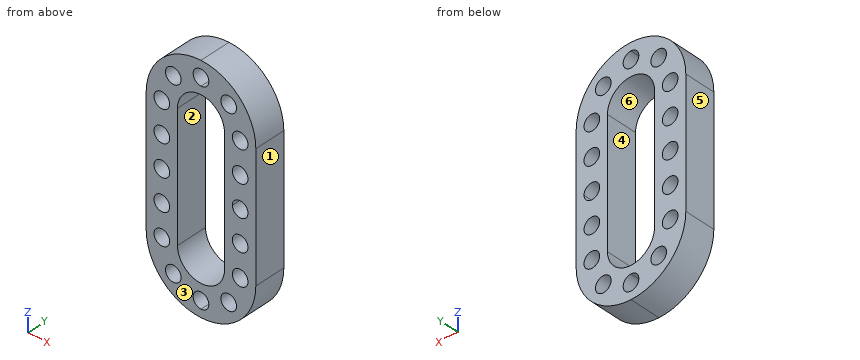
```python
from build123d import *
from build123d import SkipClean  # not in build123d's __all__

# Parameters (mm, degrees)
F0_R     = 5
F1_DEPTH = 20


with BuildPart() as f1:
    # F0 (on Front) → F1 (new body)
    with BuildSketch(Plane.XZ):
        with BuildLine():
            ThreePointArc((-15, 40), (-10.6066017178, 50.6066017178), (0, 55))
            Line((0, 55), (0.0401919294, 60.0001615417))
            ThreePointArc((0.0401919294, 60.0001615417), (-4.9999596144, 64.979903873), (0, 70))
            Line((0, 70), (0, 75))
            ThreePointArc((0, 75), (-24.7487373415, 64.7487373415), (-35, 40))
            Line((-35, 40), (-35, 0))
            Line((-35, 0), (-30, 0))
            ThreePointArc((-30, 0), (-25, 5), (-20, 0))
            Line((-20, 0), (-15, 0))
            Line((-15, 0), (-15, 40))
        make_face()
        with Locations((-25, 20)):
            Circle(F0_R, mode=Mode.SUBTRACT)
        with Locations((-25, 40)):
            Circle(F0_R, mode=Mode.SUBTRACT)
        with Locations((-17.6776695297, 57.6776695297)):
            Circle(F0_R, mode=Mode.SUBTRACT)
    extrude(amount=F1_DEPTH)

    # F2: F1 across plane


with BuildPart() as f1_1:
    add(f1.part, clean=False)
    add(f1.part.mirror(Plane.YZ), clean=False)

    # F3: F1 across plane


with BuildPart() as f1_2:
    add(f1_1.part, clean=False)
    with SkipClean():  # cleaning this boolean's faces spoils the solid; the shape is the same uncleaned
        add(f1_1.part.mirror(Plane.XY), clean=False)


solid = f1_2.part
```
For this review, take the finished solid that the model builds, in its own axes (mm). Face numbers are marked on the shaded views. A direction names the side the tool comes from. Round coordinates to 2 decimals unless told otherwise and drop trailing zeros. Order: outer loops, then holes, each group sorted by start corner. A loop starts at its lowest first (then second) coordinate and runs counter-clockwise, first axis right, second up. Notation, with made-up numbers: (18, 48.5) -> (73, 48.5) arc R9 ccw to (73, 62.5) -> close; hole circle Ø4 at (-12.75, -28). An arc over 180 degrees is marked (long way). Use a Markdown table: item, result.
Item 1: Draft analysis for pull direction X (two halves, no side actions). For the marked faces 1, 2, 3 and 4, state which applies: +X half, -X half, draft (parallel to the pull), parting line (faces both ways), or undercut.
Resolved:
| item | result |
|---|---|
| face 1 | +X half |
| face 2 | undercut |
| face 3 | draft |
| face 4 | undercut |
Item 2: Take a section at C-C (y = -9). State how many separate pieces and enclosed holes the cut face has, plus the area to 3 significant figures.
Resolved:
| item | result |
|---|---|
| separate pieces | 1 |
| enclosed holes | 17 |
| area | 5,080 mm² |
Item 3: Take a section at B-B (x = 9.5). State the section outline as (y, z) points.
Resolved:
| item | result |
|---|---|
| outline | (-20, -73.69) -> (0, -73.69) -> (0, -51.61) -> (-20, -51.61) -> close; (-20, 51.61) -> (0, 51.61) -> (0, 73.69) -> (-20, 73.69) -> close |
Item 4: For pin 1 (10 mm diameter, centred on x = 21.5, z = -14, fed in from +Y); pin 2 (12 mm diameter, centred on x = -27.5, y = -12, fed in from +Z); pin 3 (2 mm diameter, centred on x = -13.5, y = -14, fed in from -Z); pin 4 (3 mm diameter, centred on x = 4, y = -16.5, fed in from +Z), all flat-tipped, find the tip position at first contact; note any pin that passes through.
Resolved:
| item | result |
|---|---|
| pin 1 | stops at y = 0 |
| pin 2 | stops at z = 67.62 |
| pin 3 | stops at z = -72.69 |
| pin 4 | stops at z = 74.91 |
Item 5: Take a section at A-A (z = -6.5). State the section outline as (x, y) points.
Resolved:
| item | result |
|---|---|
| outline | (-35, -20) -> (-15, -20) -> (-15, 0) -> (-35, 0) -> close; (15, -20) -> (35, -20) -> (35, 0) -> (15, 0) -> close |
Item 6: For line 1 along X through (y, z) = (-6.75, -20); line 2 along X through (y, z) = (-5, -58); line 3 along X through (y, z) = (-2, -14), list the stretches that pass through material, from the lowest coordinate up. Write a range as [from, to].
Resolved:
| item | result |
|---|---|
| line 1 | x = [-35, -30], [-20, -15], [15, 20], [30, 35] |
| line 2 | x = [-30.02, -22.67], [-12.69, 12.69], [22.67, 30.02] |
| line 3 | x = [-35, -15], [15, 35] |
Item 7: Machinability: for the marked faces 5 and 6, which of the approach directions +Z, -Z, +X, -X, +Y, -Y give a long, thin tool a straight path to every point of the face, cutting with its end or side? Answer none if there is none.
Resolved:
| item | result |
|---|---|
| face 5 | +Z, -Z, -X, +Y, -Y |
| face 6 | +Y, -Y |
Item 8: Take a section at D-D (x = 25). State the section outline as (y, z) points.
Resolved:
| item | result |
|---|---|
| outline | (-20, -64.49) -> (0, -64.49) -> (0, -45) -> (-20, -45) -> close; (-20, -35) -> (0, -35) -> (0, -25) -> (-20, -25) -> close; (-20, -15) -> (0, -15) -> (0, -5) -> (-20, -5) -> close; (-20, 5) -> (0, 5) -> (0, 15) -> (-20, 15) -> close; (-20, 25) -> (0, 25) -> (0, 35) -> (-20, 35) -> close; (-20, 45) -> (0, 45) -> (0, 64.49) -> (-20, 64.49) -> close |
